Autodesk Inventor part; units mm, degrees
ref_plane "YZ Plane" through (0, 0, 0) normal (1, 0, 0) x (0, 1, 0)
ref_plane "XZ Plane" through (0, 0, 0) normal (0, 1, 0) x (-1, 0, 0)
ref_plane "XY Plane" through (0, 0, 0) normal (0, 0, 1) x (1, 0, 0)
sketch "Sketch1" plane through (0, 0, 0) normal (0, 1, 0) x (-1, 0, 0)
  line L0 (12.7, 12.7) -> (-12.7, 12.7)
  line L1 (-12.7, 12.7) -> (-12.7, -12.7)
  line L2 (-12.7, -12.7) -> (12.7, -12.7)
  line L3 (12.7, -12.7) -> (12.7, 12.7)
  line L4 (-9.525, 9.525) -> (9.525, 9.525)
  line L5 (9.525, 9.525) -> (9.525, -9.525)
  line L6 (9.525, -9.525) -> (-9.525, -9.525)
  line L7 (-9.525, -9.525) -> (-9.525, 9.525)
  point P0 (0, 0)
  point P1 (12.7, 0)
  point P2 (0, -12.7)
  dimension "d0" = 25.4
  dimension "d1" = 25.4
  dimension "d2" = 3.175
extrude "Extrusion1" add sketch "Sketch1" along normal blind 736.6
sketch "Sketch2" plane through (-12.7, 0, 12.7) normal (0, 0, 1) x (1, 0, 0)
  line L0 (0, 736.6) -> (25.4, 736.6)
  line L1 (0, 0) -> (25.4, 0)
  point P0 (12.7, 0)
  point P1 (12.7, 12.7)
  point P2 (12.7, 723.9)
  point P3 (12.7, 368.3)
  dimension "d5" = 12.7
  dimension "d6" = 12.7
  dimension "d7" = 368.3
hole "Hole1" at (0, 12.7, 12.7) at (0, 723.9, 12.7) at (0, 368.3, 12.7) direction (0, 0, -1) diameter 12.7 end through all
sketch "Sketch3" plane through (-12.7, 0, 12.7) normal (0, 0, 1) x (1, 0, 0)
  line L0 (21.6869, 114.0639) -> (21.6869, 96.9638) construction
  line L1 (21.6869, 96.9638) -> (5.8083, 96.9638) construction
  line L2 (5.8083, 96.9638) -> (5.8083, 114.0639) construction
  line L3 (5.8083, 114.0639) -> (21.6869, 114.0639) construction
  point P0 (12.7, 0)
equation "\"d0\" = Tube_size"
equation "\"d1\" = Tube_size"
equation "\"d2\" = Wall_Thickness"
equation "\"d3\" = Bar1_1_Length"
equation "\"d8\" = Pin_Size"
equation "\"Bar1_1_Length\" = 736.6"
equation "\"Tube_size_1\" = 25.4"
equation "\"Wall_Thickness_1\" = 3.175"
equation "\"Lower_Pivit_Offset_FromEdge\" = 12.7"
equation "\"Uper_Pivit_Offset_FromEdge\" = 12.7"
equation "\"Bar1_1_Center_Pivit_Offset_FromEdge\" = 368.3"
equation "\"Bar1_2_Length\" = 736.6"
equation "\"Bar2_1_Length\" = 736.6"
equation "\"Bar2_2_Length\" = 736.6"
equation "\"Bar3_1_Length\" = 736.6"
equation "\"Bar3_2_Length\" = 736.6"
equation "\"Tube_size\" = 25.4"
equation "\"Wall_Thickness\" = 3.175"
equation "\"Bar1_2_Center_Pivit_Offset_FromEdge\" = 368.3"
equation "\"Bar2_1_Center_Pivit_Offset_FromEdge\" = 368.3"
equation "\"Bar2_2_Center_Pivit_Offset_FromEdge\" = 368.3"
equation "\"Bar3_1_Center_Pivit_Offset_FromEdge\" = 368.3"
equation "\"Bar4_2_Center_Pivit_Offset_FromEdge\" = 355.6"
equation "\"Pin_Size\" = 12.7"
equation "\"Bar3_2_Center_Pivit_Offset_FromEdge\" = 368.3"
properties part number "2018 Bar1_1"
Could you check a few things on this model? Use its own coordinates, in mm. A direction names the side the tool comes from. Coordinates: 2 decimals unless noted, no trailing zeros. Loops run counter-clockwise (first coordinate to the right, second up) from the corner with the lowest first, then second, coordinate; pieces in that order, holes last. Notation, with made-up numbers: M -27.5,68 L -19.5,68 A18 cw -19.5,95 Z; hole C 14,63.25 d8. An arc over 180 degrees is marked long. Put each result on its own line as item: value. Start each with the question number.
(1) Suppose I cut it at B-B on x = 0. Count the separate pieces of the cut face and the enclosed holes in it, then the cut area to 3 significant figures.
(2) Will this pin go through, and if not, where does the flat tip stop? P1, Ø11.5, axis at x = 0, y = 12.7, coming from the +Z side.
(3) I need wall thicknesses on line 1 (Y direction, x = 0, z = -10.3); line 2 (Z direction, x = 3.75, y = 613) (3 decimals); line 3 (X direction, y = 723.9, z = -11.15). Which ranges of each line are inside material? Lowest first, please. Write a range as from..to.
(4) For faces 4 (the face through (9.525, 363, 0)), 5 (the face through (2.432, 362.434, -11.135)), which set-ups out of +Z, -Z, +X, -X, +Y, -Y let a thin tool reach every point of the face, with its end or its side?
(5) Thinking about a two-plate mould opening in Z: for faces 1 (the face through (-5, 363, -12.7)), 2 (the face through (-4, 363, 9.525)), 3 (the face through (-0.279, 730.244, -11.135)), which applies, pulls with the +Z half, pulls with the -Z half, needs draft (parallel to the pull), parting line crosses it, or undercut?
(6) Suppose I cut it at A-A on y = 368.3. Please give me the cut outline in (x, z) (3 decimals), then the cut area to 3 significant figures.
Solutions:
1. separate pieces: 8
1. enclosed holes: 0
1. area: 4,440 mm2
2. P1: passes through
3. line 1: y = 0..6.35, 19.05..361.95, 374.65..717.55, 730.25..736.6
3. line 2: z = -12.7..-9.525, 9.525..12.7
3. line 3: x = -12.7..-6.35, 6.35..12.7
4. face 4: +Y, -Y
4. face 5: +Z, -Z
5. face 1: pulls with the -Z half
5. face 2: undercut
5. face 3: needs draft
6. outline: M -12.7,-12.7 L -6.35,-12.7 L -6.35,-9.525 L -9.525,-9.525 L -9.525,9.525 L -6.35,9.525 L -6.35,12.7 L -12.7,12.7 Z; M 6.35,-12.7 L 12.7,-12.7 L 12.7,12.7 L 6.35,12.7 L 6.35,9.525 L 9.525,9.525 L 9.525,-9.525 L 6.35,-9.525 Z
6. area: 202 mm2
